Autodesk Inventor part; units mm, degrees
ref_plane "YZ Plane" through (0, 0, 0) normal (1, 0, 0) x (0, 1, 0)
ref_plane "XZ Plane" through (0, 0, 0) normal (0, 1, 0) x (-1, 0, 0)
ref_plane "XY Plane" through (0, 0, 0) normal (0, 0, 1) x (1, 0, 0)
sketch "Sketch1" plane through (0, 0, 0) normal (0, 1, 0) x (-1, 0, 0)
  circle A0 centre (60, 0) radius 1.5
  circle A1 centre (0, -60) radius 1.5
  circle A2 centre (-60, 0) radius 1.5
  circle A3 centre (0, 60) radius 1.5
  arc A4 (60, 16) -> (60, -16) centre (60, 0) ccw
  arc A5 (16, -60) -> (-16, -60) centre (0, -60) ccw
  arc A6 (-60, -16) -> (-60, 16) centre (-60, 0) ccw
  arc A7 (-16, 60) -> (16, 60) centre (0, 60) ccw
  circle A8 centre (0, 0) radius 120
  line L0 (16, 60) -> (16, 86.1626)
  line L1 (-16, 60) -> (-16, 86.1626)
  line L2 (-60, 16) -> (-86.1626, 16)
  line L3 (-60, -16) -> (-86.1626, -16)
  line L4 (-16, -60) -> (-16, -86.1626)
  line L5 (16, -60) -> (16, -98.7117)
  line L6 (60, 16) -> (86.1626, 16)
  line L7 (60, -16) -> (86.1626, -16)
  arc A9 (-28.8889, 95.7363) -> (-95.7363, 28.8889) centre (0, 0) ccw
  arc A10 (-95.7363, -28.8889) -> (-28.8889, -95.7363) centre (0, 0) ccw
  arc A11 (16, -98.7117) -> (95.7363, -28.8889) centre (0, 0) ccw
  arc A12 (95.7363, 28.8889) -> (28.8889, 95.7363) centre (0, 0) ccw
  arc A13 (28.8889, 95.7363) -> (16, 86.1626) centre (26, 86.1626) ccw
  arc A14 (86.1626, 16) -> (95.7363, 28.8889) centre (86.1626, 26) ccw
  arc A15 (95.7363, -28.8889) -> (86.1626, -16) centre (86.1626, -26) ccw
  arc A16 (-28.8889, -95.7363) -> (-16, -86.1626) centre (-26, -86.1626) ccw
  arc A17 (-86.1626, -16) -> (-95.7363, -28.8889) centre (-86.1626, -26) ccw
  arc A18 (-95.7363, 28.8889) -> (-86.1626, 16) centre (-86.1626, 26) ccw
  arc A19 (-16, 86.1626) -> (-28.8889, 95.7363) centre (-26, 86.1626) ccw
  line L8 (0, 0) -> (110, 0) construction
  circle A20 centre (95.8524, 53.966) radius 1.5
  circle A21 centre (56.0276, 94.6621) radius 1.5
  circle A22 centre (1.1903, 109.9936) radius 1.5
  circle A23 centre (-53.966, 95.8524) radius 1.5
  circle A24 centre (-94.6621, 56.0276) radius 1.5
  circle A25 centre (-109.9936, 1.1903) radius 1.5
  circle A26 centre (-95.8524, -53.966) radius 1.5
  circle A27 centre (-56.0276, -94.6621) radius 1.5
  circle A28 centre (-1.1903, -109.9936) radius 1.5
  circle A29 centre (53.966, -95.8524) radius 1.5
  circle A30 centre (94.6621, -56.0276) radius 1.5
  circle A31 centre (109.9936, -1.1903) radius 1.5
  point P0 (16, 98.7117)
  point P1 (-16, 98.7117)
  point P2 (-98.7117, 16)
  point P3 (-98.7117, -16)
  point P4 (-16, -98.7117)
  point P5 (98.7117, 16)
  point P6 (98.7117, -16)
  dimension "d1" = 3
  dimension "d2" = 3
  dimension "d3" = 3
  dimension "d4" = 3
  dimension "d5" = 32
  dimension "d6" = 32
  dimension "d7" = 32
  dimension "d8" = 32
  dimension "d14" = 10
  dimension "d17" = 3
  dimension "d20" = 360
extrude "Extrusion1" add sketch "Sketch1" along normal blind 2
properties part number "shell top bracket"
Work out the finished part from the listing and answer in its coordinate system (mm). A direction names the side the tool comes from. Coordinates: 2 decimals unless noted, no trailing zeros. Write each loop counter-clockwise with the first axis right and the second up, starting at its lowest first coordinate (ties: lowest second). Pieces come first, ordered by that corner, then holes.
Q1. A cutting plane is placed at A-A, the plane x = 12. Give the vertices of the cut face in (y, z).
Q2. Determine the mould class of faces 1 (the face through (1, 2, 45)), 2 (the face through (119.884, 0.986, -5.276)), 3 (the face through (20.142, 0.986, 94.267)), 4 (the face through (-44, 1, 0)) for opening direction X: released by +X, released by -X, zero draft, split by the parting line, or undercut.
Q3. Each of these flat-tipped pins is pushed along its axis until it touches: pin 1 Ø3.5 at (x, z) = (-95.85, 53.97) entering from -Y; pin 2 Ø1 at (y, z) = (1, 87.5) entering from -X; pin 3 Ø0.6 at (x, y) = (76.5, 1.5) entering from -Z; pin 4 Ø1 at (x, y) = (-58.5, 0.5) entering from +Z. Where does it stop, or does it pass through?
Q4. A cutting plane is placed at C-C, the plane x = 89. Give the vertices of the cut face in (y, z), then the cut area to 3 significant figures.
Q5. A cutting plane is placed at B-B, the plane z = -41. Give the vertices of the cut face in (x, y).
Q6. A cutting plane is placed at D-D, the plane y = 0.7. State how many separate pieces and enclosed holes the cut face has, then the cut area to 3 significant figures.
Q7. Find the intervals of material crossed by line 1 (X direction, y = 1.8, z = -68.5); line 2 (Z direction, x = 74.5, y = 0.2); line 3 (X direction, y = 0.5, z = 50.5), in increasing order.
Q8. Which of the six approach directions +Z, -Z, +X, -X, +Y, -Y give full straight-line access (tool end or side, diameter ignored) to faces 5 (the face through (19.93, 0.99, -94.11)), 6 (the face through (1, 0, 45))?
Findings below:
1. outline: (0, -119.4) - (2, -119.4) - (2, -49.42) - (0, -49.42) - close; (0, 49.42) - (2, 49.42) - (2, 119.4) - (0, 119.4) - close
2. face 1: zero draft
2. face 2: split by the parting line
2. face 3: undercut
2. face 4: undercut
3. pin 1: stops at y = 0
3. pin 2: stops at x = -82.65
3. pin 3: stops at z = -92.7
3. pin 4: stops at z = 105.05
4. outline: (0, -80.49) - (2, -80.49) - (2, -45.6) - (0, -45.6) - close; (0, -16.41) - (2, -16.41) - (2, 16.41) - (0, 16.41) - close; (0, 45.6) - (2, 45.6) - (2, 80.49) - (0, 80.49) - close
4. area: 205 mm2
5. outline: (-112.78, 0) - (-91.21, 0) - (-91.21, 2) - (-112.78, 2) - close; (91.21, 0) - (112.78, 0) - (112.78, 2) - (91.21, 2) - close
6. separate pieces: 1
6. enclosed holes: 17
6. area: 20,600 mm2
7. line 1: x = -98.53 to -72.85, -16 to 16, 72.85 to 98.53
7. line 2: z = -94.07 to -66.71, -16 to 16, 66.71 to 94.07
7. line 3: x = -108.86 to -86.31, -12.87 to 12.87, 86.31 to 108.86
8. face 5: +Y, -Y
8. face 6: +Z, -Z, +X, -X, -Y
